For this review, use the dimensioned drawing (mm, ordinates from the lowest corner) and the shaded views. A direction names the side the tool comes from. Coordinates: 2 decimals unless noted, no trailing zeros. Loops run counter-clockwise (first coordinate to the right, second up) from the corner with the lowest first, then second, coordinate; pieces in that order, holes last. Notation, with made-up numbers: (87.5, 61.5) - (140.5, 61.5) arc R9 ccw to (140.5, 65.5) - close; hole circle Ø8 at (24.5, 65). An arc over 180 degrees is marked (long way). Use one line per item in the form item = value. Start each with the question number.
(1) Add section D-D (x = 15.5). State the section outline as (y, z) points (3 decimals).
(2) For L1, parallel to X at y = 6.5, z = 3.5 (3 decimals); L2, parallel to Z at x = 38.1, y = 5; L3, parallel to Z at x = 10, y = 7.25, list the stretches that pass through material, from the lowest coordinate up.
(3) Tool access review of the marked faces 4 and 5: name each direction out of +Z, -Z, +X, -X, +Y, -Y from which nothing blocks a thin tool from reaching the whole face with its end or side.
(4) Add section C-C (x = 38.1). State the section outline as (y, z) points (3 decimals), plus the area to 3 significant figures.
(5) Clearance check with flat-ended pins moving along their axes: pin 1 Ø1 at (y, z) = (6.5, 7.5) entering from -X; pin 2 Ø1.5 at (x, y) = (19.5, 6) entering from -Z; pin 3 Ø1.8 at (x, z) = (3.175, 7.62) entering from +Y (3 decimals). State where each tip first meets the part, or that it passes through.
(6) Add section B-B (y = 5.5). State the section outline as (x, z) points (3 decimals).
(7) Add section A-A (z = 9.5). State the section outline as (x, y) points (3 decimals).
(8) The part is to be moulded in two halves that separate along X. For the marked faces 1, 2 and 3, say which applies: pulls with the +X half, pulls with the -X half, needs draft (parallel to the pull), parting line crosses it, or undercut.
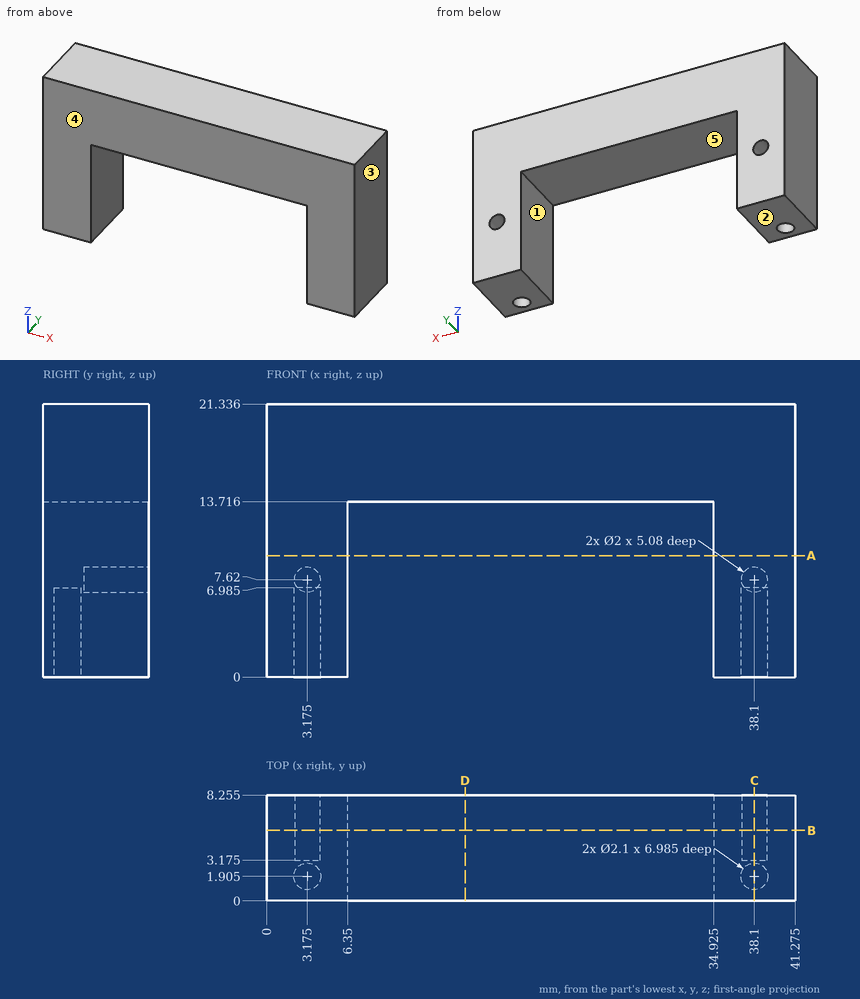
Computed values:
q1.outline = (0, 13.716) - (8.255, 13.716) - (8.255, 21.336) - (0, 21.336) - close
q2.L1 = 0 to 6.35, 34.925 to 41.275
q2.L2 = 0 to 6.62, 8.62 to 21.34
q2.L3 = 13.72 to 21.34
q3.face_4 = +Z, -Z, +X, -X, -Y
q3.face_5 = -Z, +Y, -Y
q4.outline = (0, 0) - (0.855, 0) - (0.855, 6.985) - (2.955, 6.985) - (2.955, 0) - (8.255, 0) - (8.255, 6.62) - (3.175, 6.62) - (3.175, 8.62) - (8.255, 8.62) - (8.255, 21.336) - (0, 21.336) - close
q4.area = 151 mm^2
q5.pin_1 = 0
q5.pin_2 = 13.72
q5.pin_3 = 3.175
q6.outline = (0, 0) - (6.35, 0) - (6.35, 13.716) - (34.925, 13.716) - (34.925, 0) - (41.275, 0) - (41.275, 21.336) - (0, 21.336) - close; hole circle Ø2 at (3.175, 7.62); hole circle Ø2 at (38.1, 7.62)
q7.outline = (0, 0) - (6.35, 0) - (6.35, 8.255) - (0, 8.255) - close; (34.925, 0) - (41.275, 0) - (41.275, 8.255) - (34.925, 8.255) - close
q8.face_1 = undercut
q8.face_2 = needs draft
q8.face_3 = pulls with the +X half
